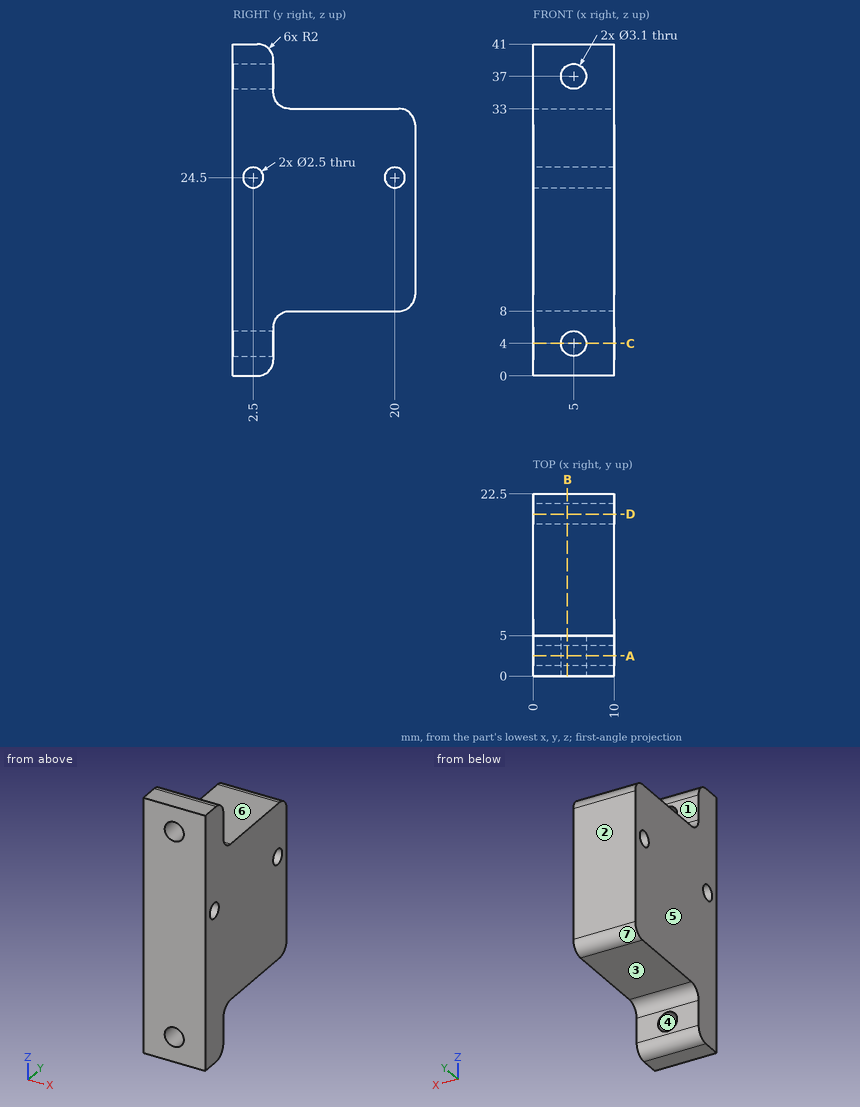
Could you check a few things on this drawing? It's one solid part, dimensions in mm from its lowest x, y, z. A direction names the side the tool comes from. Coordinates: 2 decimals unless noted, no trailing zeros. Order: outer loops, then holes, each group sorted by start corner. A loop starts at its lowest first (then second) coordinate and runs counter-clockwise, first axis right, second up.
1. If we section it at D-D (y = 20): Please give me the cut outline in (x, z), then the cut area to 3 significant figures.
2. If we section it at B-B (x = 4.25): Please give me the cut outline in (y, z).
3. Thinking about a two-plate mould opening in Z: for the marked faces 4, 5, 6 and 7, which applies, +Z half, -Z half, draft (parallel to the pull), parting line (faces both ways), or undercut?
4. I need wall thicknesses on line 1 (Y direction, x = 2.5, z = 24.5); line 2 (Z direction, x = 5, y = 2.65); line 3 (X direction, y = 1.15, z = 4). Which ranges of each line are inside material? Lowest first, please.
5. For the marked faces 1, 2 and 3, which set-ups out of +Z, -Z, +X, -X, +Y, -Y let a thin tool reach every point of the face, with its end or its side?
6. If we section it at C-C (z = 4): Please give me the cut outline in (x, y), then the cut area to 3 significant figures.
7. I'm going to push flat-ended pins straight in: pin 1 (5 mm diameter, centred on x = 7.5, y = 11.5, fed in from +Z); pin 2 (2 mm diameter, centred on x = 4, z = 38, fed in from +Y); pin 3 (5 mm diameter, centred on x = 7.5, z = 5, fed in from +Y); pin 4 (1.9 mm diameter, centred on x = 5, z = 37, fed in from +Y). Where does each tip first touch, or does it pass through?
8. If we section it at A-A (y = 2.5): Please give me the cut outline in (x, z), then the cut area to 3 significant figures.
Entries:
1. outline: (0, 8) - (10, 8) - (10, 23.25) - (0, 23.25) - close; (0, 25.75) - (10, 25.75) - (10, 33) - (0, 33) - close
1. area: 225 mm2
2. outline: (0, 0) - (3, 0) arc R2 ccw to (5, 2) - (5, 2.64) - (0, 2.64) - close; (0, 5.36) - (5, 5.36) - (5, 6) arc R2 cw to (7, 8) - (20.5, 8) arc R2 ccw to (22.5, 10) - (22.5, 31) arc R2 ccw to (20.5, 33) - (7, 33) arc R2 cw to (5, 35) - (5, 35.64) - (0, 35.64) - close; (0, 38.36) - (5, 38.36) - (5, 39) arc R2 ccw to (3, 41) - (0, 41) - close; hole circle Ø2.5 at (2.5, 24.5); hole circle Ø2.5 at (20, 24.5)
3. face 4: undercut
3. face 5: draft
3. face 6: +Z half
3. face 7: -Z half
4. line 1: y = 0 to 1.25, 3.75 to 18.75, 21.25 to 22.5
4. line 2: z = 0 to 2.45, 5.55 to 23.26, 25.74 to 35.45, 38.55 to 41
4. line 3: x = 0 to 3.45, 6.55 to 10
5. face 1: +Z, +X, -X, +Y
5. face 2: +Z, -Z, +X, -X, +Y
5. face 3: -Z, +X, -X, +Y
6. outline: (0, 0) - (3.45, 0) - (3.45, 5) - (0, 5) - close; (6.55, 0) - (10, 0) - (10, 5) - (6.55, 5) - close
6. area: 34.5 mm2
7. pin 1: stops at z = 33
7. pin 2: stops at y = 5
7. pin 3: stops at y = 5.68
7. pin 4: passes through
8. outline: (0, 0) - (10, 0) - (10, 23.25) - (0, 23.25) - close; (0, 25.75) - (10, 25.75) - (10, 41) - (0, 41) - close; hole circle Ø3.1 at (5, 4); hole circle Ø3.1 at (5, 37)
8. area: 370 mm2
